```python
from build123d import *

# Parameters (mm, degrees)
F0_R     = 3.55
F1_DEPTH = 4.5
F2_W     = 51.5
F2_H     = 62.85
F3_DEPTH = 4.501
F4_R     = 1.6
F5_DEPTH = 4.501
F6_R     = 4
F7_DEPTH = 2.5


with BuildPart() as f1:
    # F0 (on Top) → F1 (new body)
    with BuildSketch(Plane.XY):
        with BuildLine():
            ThreePointArc((-72.175, -48), (-69.538961, -54.363961), (-63.175, -57))
            Line((-63.175, -57), (-46, -57))
            ThreePointArc((-46, -57), (-42.5, -53.5), (-39, -57))
            Line((-39, -57), (-3.5, -57))
            ThreePointArc((-3.5, -57), (0, -53.5), (3.5, -57))
            Line((3.5, -57), (39, -57))
            ThreePointArc((39, -57), (42.5, -53.5), (46, -57))
            Line((46, -57), (63.175, -57))
            ThreePointArc((63.175, -57), (69.538961, -54.363961), (72.175, -48))
            Line((72.175, -48), (72.175, -38.175))
            Line((72.175, -38.175), (73, -38.175))
            ThreePointArc((73, -38.175), (79.363961, -35.538961), (82, -29.175))
            Line((82, -29.175), (82, -3.5))
            ThreePointArc((82, -3.5), (78.5, 0), (82, 3.5))
            Line((82, 3.5), (82, 29.175))
            ThreePointArc((82, 29.175), (79.363961, 35.538961), (73, 38.175))
            Line((73, 38.175), (72.175, 38.175))
            Line((72.175, 38.175), (72.175, 48))
            ThreePointArc((72.175, 48), (69.538961, 54.363961), (63.175, 57))
            Line((63.175, 57), (46, 57))
            ThreePointArc((46, 57), (42.5, 53.5), (39, 57))
            Line((39, 57), (3.5, 57))
            ThreePointArc((3.5, 57), (0, 53.5), (-3.5, 57))
            Line((-3.5, 57), (-39, 57))
            ThreePointArc((-39, 57), (-42.5, 53.5), (-46, 57))
            Line((-46, 57), (-63.175, 57))
            ThreePointArc((-63.175, 57), (-69.538961, 54.363961), (-72.175, 48))
            Line((-72.175, 48), (-72.175, 38.175))
            Line((-72.175, 38.175), (-73, 38.175))
            ThreePointArc((-73, 38.175), (-79.363961, 35.538961), (-82, 29.175))
            Line((-82, 29.175), (-82, 3.5))
            ThreePointArc((-82, 3.5), (-78.5, 0), (-82, -3.5))
            Line((-82, -3.5), (-82, -29.175))
            ThreePointArc((-82, -29.175), (-79.363961, -35.538961), (-73, -38.175))
            Line((-73, -38.175), (-72.175, -38.175))
            Line((-72.175, -38.175), (-72.175, -48))
        make_face()
        with Locations((-66, -45.5)):
            Circle(F0_R, mode=Mode.SUBTRACT)
        with Locations((52, -45.5)):
            Circle(F0_R, mode=Mode.SUBTRACT)
        with Locations((66, -45.5)):
            Circle(F0_R, mode=Mode.SUBTRACT)
        with Locations((-66, 45.5)):
            Circle(F0_R, mode=Mode.SUBTRACT)
        with Locations((52, 45.5)):
            Circle(F0_R, mode=Mode.SUBTRACT)
        with Locations((66, 45.5)):
            Circle(F0_R, mode=Mode.SUBTRACT)
    extrude(amount=F1_DEPTH)

    # F2 (on face) → F3 (cut, through all)
    with BuildSketch(Plane.XY.offset(4.5)):
        with Locations((42.425, -3.575)):
            Rectangle(F2_W, F2_H)
    extrude(amount=-F3_DEPTH, mode=Mode.SUBTRACT)

    # F4 (on face) → F5 (cut, through all)
    with BuildSketch(Plane.XY.offset(4.5)):
        with Locations((-54.6625, 45)):
            Circle(F4_R)
        with Locations((-54.6625, 33)):
            Circle(F4_R)
        with Locations((-54.6625, 21)):
            Circle(F4_R)
        with Locations((-54.6625, 9)):
            Circle(F4_R)
        with Locations((-54.6625, -3)):
            Circle(F4_R)
        with Locations((-54.6625, -15)):
            Circle(F4_R)
        with Locations((-54.6625, -27)):
            Circle(F4_R)
        with Locations((-54.6625, -39)):
            Circle(F4_R)
        with Locations((-10.6625, 38)):
            Circle(F4_R)
        with Locations((-10.6625, 26)):
            Circle(F4_R)
        with Locations((-10.6625, 14)):
            Circle(F4_R)
        with Locations((-10.6625, 2)):
            Circle(F4_R)
        with Locations((-10.6625, -10)):
            Circle(F4_R)
        with Locations((-10.6625, -22)):
            Circle(F4_R)
        with Locations((-10.6625, -34)):
            Circle(F4_R)
        with Locations((-10.6625, -46)):
            Circle(F4_R)
        with Locations((-32.6625, 41.5)):
            Circle(F4_R)
        with Locations((-32.6625, 29.5)):
            Circle(F4_R)
        with Locations((-32.6625, 17.5)):
            Circle(F4_R)
        with Locations((-32.6625, 5.5)):
            Circle(F4_R)
        with Locations((-32.6625, -6.5)):
            Circle(F4_R)
        with Locations((-32.6625, -18.5)):
            Circle(F4_R)
        with Locations((-32.6625, -30.5)):
            Circle(F4_R)
        with Locations((-32.6625, -42.5)):
            Circle(F4_R)
    extrude(amount=-F5_DEPTH, mode=Mode.SUBTRACT)

    # F6 (on face) → F7 (cut)
    with BuildSketch(Plane(origin=(0, 0, 0), x_dir=(1, 0, 0), z_dir=(0, 0, -1))):
        with Locations((-10.6625, 46)):
            Circle(F6_R)
        with Locations((-10.6625, 34)):
            Circle(F6_R)
        with Locations((-10.6625, 22)):
            Circle(F6_R)
        with Locations((-10.6625, 10)):
            Circle(F6_R)
        with Locations((-10.6625, -2)):
            Circle(F6_R)
        with Locations((-10.6625, -14)):
            Circle(F6_R)
        with Locations((-10.6625, -26)):
            Circle(F6_R)
        with Locations((-54.6625, 39)):
            Circle(F6_R)
        with Locations((-54.6625, 27)):
            Circle(F6_R)
        with Locations((-54.6625, 15)):
            Circle(F6_R)
        with Locations((-54.6625, 3)):
            Circle(F6_R)
        with Locations((-54.6625, -9)):
            Circle(F6_R)
        with Locations((-54.6625, -21)):
            Circle(F6_R)
        with Locations((-54.6625, -33)):
            Circle(F6_R)
        with Locations((-10.6625, -38)):
            Circle(F6_R)
        with Locations((-54.6625, -45)):
            Circle(F6_R)
        with Locations((-32.6625, 42.5)):
            Circle(F6_R)
        with Locations((-32.6625, 30.5)):
            Circle(F6_R)
        with Locations((-32.6625, 18.5)):
            Circle(F6_R)
        with Locations((-32.6625, 6.5)):
            Circle(F6_R)
        with Locations((-32.6625, -5.5)):
            Circle(F6_R)
        with Locations((-32.6625, -17.5)):
            Circle(F6_R)
        with Locations((-32.6625, -29.5)):
            Circle(F6_R)
        with Locations((-32.6625, -41.5)):
            Circle(F6_R)
    extrude(amount=-F7_DEPTH, mode=Mode.SUBTRACT)


solid = f1.part
```
Check sheet for the modelled part. Datum: model origin and axes. Units: mm. A direction names the side the tool comes from. Round coordinates to 2 decimals unless told otherwise and drop trailing zeros. Loops run counter-clockwise (first coordinate to the right, second up) from the corner with the lowest first, then second, coordinate; pieces in that order, holes last. Notation, with made-up numbers: (52.25, 70) - (79.25, 70) arc R23 ccw to (79.25, 104) - close; hole circle Ø10 at (-26, 17.5). An arc over 180 degrees is marked (long way). Answer as a JSON object with one key per item and string values. Group by question number.
Q1. Scan lines: line 1 along Y through (x, z) = (38, 1.8); line 2 along Y through (x, z) = (43, 3.05); line 3 along X through (y, z) = (-24, 1.05) (3 decimals). Record each from-to range of solid material in increasing order. Write a range as [from, to].
Q2. Sectioned sample at B-B, the plane x = 66. Enter the section's corners in (y, z), plus the area to 3 significant figures.
Q3. Sectioned sample at C-C, the plane z = 1.15. Count the separate pieces of the cut face and the enclosed holes in it, plus the area to 3 significant figures.
Q4. Mould release check, pull along Y, two halves, no side actions. Record for faces 3 (the face through (-69.6, -54.3, 2.2)), 4 (the face through (-72.175, -43, 2)), 5 (the face through (-8.9, 37.9, 2.5)): released by +Y, released by -Y, zero draft, split by the parting line, or undercut.
Q5. Sectioned sample at A-A, the plane x = 42.5. Enter the section's corners in (y, z), plus the area to 3 significant figures.
Q6. Set-up check for faces 1 (the face through (-53.924, 31.581, 3.514)), 2 (the face through (-52.51, 29.63, 1.23)): record each of +Z, -Z, +X, -X, +Y, -Y from which the full face is reachable in a straight line by a thin tool's end or side.
Q7. Gauge pin test, flat ends, axial feed: P1, Ø2.5, axis at x = -11, y = -24, coming from the -Z side; P2, Ø6.5, axis at x = -54.5, y = 31.5, coming from the -Z side; P3, Ø1.3, axis at y = -42, z = 2.5, coming from the -X side (3 decimals). Record the tip position at first contact, or that the pin passes through.
Solution:
{
 "1": {"line 1": "y = [-57, -35], [27.85, 57]", "line 2": "y = [-53.54, -35], [27.85, 53.54]", "line 3": "x = [-82, -57.308], [-52.017, -14.127], [-7.198, 16.675], [68.175, 82]"},
 "2": {"outline": "(-56.55, 0) - (-49.05, 0) - (-49.05, 4.5) - (-56.55, 4.5) - close; (-41.95, 0) - (-35, 0) - (-35, 4.5) - (-41.95, 4.5) - close; (27.85, 0) - (41.95, 0) - (41.95, 4.5) - (27.85, 4.5) - close; (49.05, 0) - (56.55, 0) - (56.55, 4.5) - (49.05, 4.5) - close", "area": "162 mm²"},
 "3": {"separate pieces": "1", "enclosed holes": "31", "area": "13,000 mm²"},
 "4": {"face 3": "released by -Y", "face 4": "zero draft", "face 5": "undercut"},
 "5": {"outline": "(-53.5, 0) - (-35, 0) - (-35, 4.5) - (-53.5, 4.5) - close; (27.85, 0) - (53.5, 0) - (53.5, 4.5) - (27.85, 4.5) - close", "area": "199 mm²"},
 "6": {"face 1": "+Z, -Z", "face 2": "-Z"},
 "7": {"P1": "stops at z = 2.5", "P2": "stops at z = 0", "P3": "stops at x = -72.175"}
}
